from build123d import *

# Parameters (mm, degrees)
F0_W        = 60
F0_H        = 50
F1_DEPTH    = 50
F2_W        = 15
F2_H        = 50
F5_DEPTH    = 13
F6_T1_DEPTH = 138.4834301858
F7_R        = 5


# Not quite as in the source:
# - a fillet or chamfer that OpenCascade refuses, or shapes differently, is made with other operations: its cross-section is extruded or revolved along the edge and cut away or added


with BuildPart() as f1:
    # F0 (on Top) → F1 (new body)
    with BuildSketch(Plane.XY):
        with Locations((30, -25)):
            Rectangle(F0_W, F0_H)
    extrude(amount=F1_DEPTH)

    # F2 (on Right) → F3 (revolve, cut)
    with BuildSketch(Plane.YZ):
        with Locations((-7.5, 25)):
            Rectangle(F2_W, F2_H)
        with BuildLine():
            Line((-30, 50), (-40, 50))
            ThreePointArc((-40, 50), (-35, 45), (-30, 50))
        make_face()
    revolve(axis=Axis((0, 0, 25), (0, 0, 1)), mode=Mode.SUBTRACT)

    # F4 (on face) → F5 (cut)
    with BuildSketch(Plane.XZ.offset(50)):
        with BuildLine():
            Line((60, 50), (35, 50))
            Line((35, 50), (35, 45))
            ThreePointArc((35, 45), (37.9289321881, 37.9289321881), (45, 35))
            Line((45, 35), (60, 35))
            Line((60, 35), (60, 50))
        make_face()
    extrude(amount=-F5_DEPTH, mode=Mode.SUBTRACT)

    # F6: chamfer of 20 x 11.5470053838 on 1 edges, made by hand

    # F6_s2 → F6_t1 (cut)
    with BuildSketch(Plane.XZ.offset(-36.7417150929)):
        Polygon((20, 0), (0, 11.5470053838), (0, 0), align=None)
    extrude(amount=F6_T1_DEPTH, mode=Mode.SUBTRACT)

    # F7
    f7_edges = [f1.edges().sort_by_distance(p)[0] for p in [
        (60, 0, 25),
        (60, -25, 0),
        (40, 0, 0),
    ]]
    fillet(f7_edges, radius=F7_R)


solid = f1.part
Verification items for the finished model (mm, model axes). A direction names the side the tool comes from. Round coordinates to 2 decimals unless told otherwise and drop trailing zeros. Write each loop counter-clockwise with the first axis right and the second up, starting at its lowest first coordinate (ties: lowest second). Pieces come first, ordered by that corner, then holes.
(1) Section check C-C (z = 32.5). Enter the section's corners in (x, y).
Returned:
outline: (0, -50) - (60, -50) - (60, -5) arc R5 ccw to (55, 0) - (15, 0) arc R15 cw to (0, -15) - close
(2) Material ranges on line 1 (Y direction, x = 50, z = 48); line 2 (Z direction, x = 20, y = -28.5); line 3 (Y direction, x = 57, z = 14), recorded low to high.
Returned:
line 1: y = -37 to 0
line 2: z = 0 to 45
line 3: y = -50 to -0.42
(3) Depth check by flat-ended pin: pin 1 Ø4.5 at (x, z) = (50.5, 45) entering from -Y; pin 2 Ø5.5 at (y, z) = (-41.5, 48) entering from +X; pin 3 Ø6.5 at (x, y) = (53, -46) entering from +Z. Enter the tip coordinate at first touch or a pass-through.
Returned:
pin 1: stops at y = -37
pin 2: stops at x = 35
pin 3: stops at z = 35
(4) Section check D-D (z = 9). Enter the section's corners in (x, y), plus the area to 3 significant figures.
Returned:
outline: (4.41, -50) - (60, -50) - (60, -5) arc R5 ccw to (55, 0) - (15, 0) arc R15 cw to (4.41, -14.34) - close
area: 2,660 mm2
(5) Access from +Z, -Z, +X, -X, +Y, -Y to the whole of each face (thin tool, end or side, straight path). Record for faces 1 (the flat face through (52, -44, 35)), 2 (the flat face through (36, -30, 50)).
Returned:
face 1: +Z, +X, -Y
face 2: +Z, +X, -X, +Y, -Y
(6) Section check B-B (y = -43.5). Enter the section's corners in (x, z), plus the area to 3 significant figures.
Returned:
outline: (0, 11.55) - (20, 0) - (55, 0) arc R5 ccw to (60, 5) - (60, 35) - (45, 35) arc R10 cw to (35, 45) - (35, 50) - (0, 50) - close
area: 2,530 mm2
(7) Section check A-A (z = 47.5). Enter the section's corners in (x, y), plus the area to 3 significant figures.
Returned:
outline: (0, -50) - (35, -50) - (35, -37) - (60, -37) - (60, -5) arc R5 ccw to (55, 0) - (39.33, 0) arc R39.33 cw to (0, -39.33) - close; (0, -30.67) arc R30.67 ccw to (30.67, 0) - (15, 0) arc R15 cw to (0, -15) - close
area: 2,020 mm2
